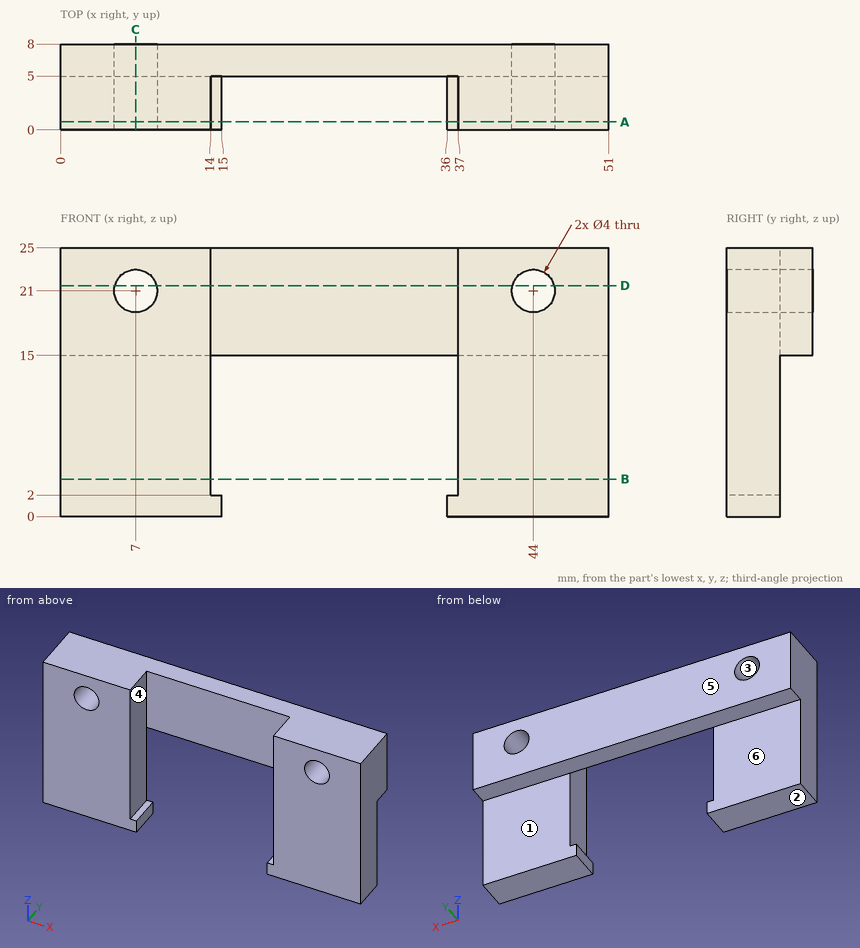
Input: dimensioned drawing with shaded views. Units: mm. Origin: part minimum x, y, z. A direction names the side the tool comes from. Give positions to 0.01 mm unless a question says otherwise; leave off trailing zeros. Write each loop counter-clockwise with the first axis right and the second up, starting at its lowest first coordinate (ties: lowest second). Pieces come first, ordered by that corner, then holes.
1. Section query C-C, the plane x = 7. Return loops of the section in (y, z).
2. Section query B-B, the plane z = 3.5. Return loops of the section in (x, y).
3. Section query D-D, the plane z = 21.5. Return loops of the section in (x, y), then the cut area to 3 significant figures.
4. Reachability of the marked faces 4, 5 and 6 from +Z, -Z, +X, -X, +Y, -Y: full face, straight path, thin tool, end or side. Return the list, or none.
5. Pin query (flat end, axial travel): P1, Ø5, axis at x = 27, z = 18, coming from the -Y side; P2, Ø12, axis at x = 44, z = 4, coming from the +Y side; P3, Ø3.5, axis at x = 26.5, y = 7, coming from the -Z side. Return the tip coordinate at first contact, or that it passes through.
6. Draft query along Z for the marked faces 1, 2 and 3. Return one class per face: released by +Z, released by -Z, zero draft, split by the parting line, or undercut.
7. Line query: probe 1 along X at (y, z) = (2.5, 21); probe 2 along X at (y, z) = (5.75, 21); probe 3 along X at (y, z) = (3.75, 9.5). Output: solid intervals per line, ascending.
8. Section query A-A, the plane y = 0.75. Return loops of the section in (x, z), then the cut area to 3 significant figures.
Computed:
1. outline: (0, 0) - (5, 0) - (5, 15) - (8, 15) - (8, 19) - (0, 19) - close; (0, 23) - (8, 23) - (8, 25) - (0, 25) - close
2. outline: (0, 0) - (14, 0) - (14, 5) - (0, 5) - close; (37, 0) - (51, 0) - (51, 5) - (37, 5) - close
3. outline: (0, 0) - (5.06, 0) - (5.06, 8) - (0, 8) - close; (8.94, 0) - (14, 0) - (14, 5) - (37, 5) - (37, 0) - (42.06, 0) - (42.06, 8) - (8.94, 8) - close; (45.94, 0) - (51, 0) - (51, 8) - (45.94, 8) - close
3. area: 231 mm2
4. face 4: +Z, -Y
4. face 5: +Z, -Z, +X, -X, +Y
4. face 6: -Z, +X, -X, +Y
5. P1: stops at y = 5
5. P2: stops at y = 5
5. P3: stops at z = 15
6. face 1: zero draft
6. face 2: released by -Z
6. face 3: undercut
7. probe 1: x = 0 to 5, 9 to 14, 37 to 42, 46 to 51
7. probe 2: x = 0 to 5, 9 to 42, 46 to 51
7. probe 3: x = 0 to 14, 37 to 51
8. outline: (0, 0) - (15, 0) - (15, 2) - (14, 2) - (14, 25) - (0, 25) - close; (36, 0) - (51, 0) - (51, 25) - (37, 25) - (37, 2) - (36, 2) - close; hole circle Ø4 at (7, 21); hole circle Ø4 at (44, 21)
8. area: 679 mm2
